from build123d import *

# Parameters (mm, degrees)
PAD_DEPTH       = 80
POCKET_DEPTH    = 78
POCKET001_DEPTH = 408.7079232475
POCKET002_DEPTH = 408.4326470939
SKETCH004_W     = 433.609177
SKETCH004_H     = 149.2376851805
SKETCH004_W_2   = 114.034424
SKETCH004_H_2   = 150.6867891805
POCKET003_DEPTH = 80.001
SKETCH005_W     = 8
SKETCH005_H     = 8
POCKET004_DEPTH = 10
SKETCH006_W     = 8
SKETCH006_H     = 8
POCKET005_DEPTH = 10
SKETCH007_R     = 1.55
POCKET006_DEPTH = 12.001
POCKET007_DEPTH = 12.001
FILLET_R        = 2
FILLET001_R     = 2


with BuildPart() as part:
    # Sketch → Pad (new body)
    with BuildSketch(Plane.XY):
        Polygon((450, 0), (450, 90), (356, 87.18), (355.64, 99.18), (343.64, 98.82), (344, 86.82), (6, 76.68), (5.64, 88.6800000001), (-6.36, 88.3200000001), (-6, 76.32), (-50, 75), (-50, 0), align=None)
    extrude(amount=PAD_DEPTH)

    # Sketch001 (on Face14 of Pad) → Pocket (cut)
    with BuildSketch(Plane.XY.offset(80)):
        Polygon((-50, 15), (-50, 74), (450, 74), (450, 0), (356, 2.82), (356.3, 12.82), (344.3, 13.18), (344, 3.18), (6, 13.32), (6.3, 23.32), (-5.7, 23.68), (-6, 13.68), align=None)
    extrude(amount=-POCKET_DEPTH, mode=Mode.SUBTRACT)

    # Sketch002 (on Face26 of Pocket) → Pocket001 (cut, through all)
    with BuildSketch(Plane(origin=(355.5953641722, -10.6678609252, 0), x_dir=(0.0299865091, 0.9995503035, 0), z_dir=(0.9995503035, -0.0299865091, 0))):
        with BuildLine():
            ThreePointArc((23.4984280855, 56), (19.9988591841, 57.4495689014), (21.4484280855, 53.95))
            ThreePointArc((21.4484280855, 53.95), (17.8329435114, 41), (21.4484280855, 28.05))
            ThreePointArc((21.4484280855, 28.05), (19.9988591841, 24.5504310986), (23.4984280855, 26))
            Line((23.4984280855, 26), (23.4984280855, 56))
        make_face()
    extrude(amount=-POCKET001_DEPTH, mode=Mode.SUBTRACT)

    # Sketch003 (on Face14 of Pocket001) → Pocket002 (cut, through all)
    with BuildSketch(Plane(origin=(358.2929363573, 10.7487880907, 0), x_dir=(-0.0299865091, 0.9995503035, 0), z_dir=(0.9995503035, 0.0299865091, 0))):
        with BuildLine():
            ThreePointArc((88.470997005, 56), (84.9714281036, 57.4495689014), (86.420997005, 53.95))
            ThreePointArc((86.420997005, 53.95), (82.8055124309, 41), (86.420997005, 28.05))
            ThreePointArc((86.420997005, 28.05), (84.9714281036, 24.5504310986), (88.470997005, 26))
            Line((88.470997005, 26), (88.470997005, 56))
        make_face()
    extrude(amount=-POCKET002_DEPTH, mode=Mode.SUBTRACT)

    # Sketch004 (on Face7 of Pocket002) → Pocket003 (cut, through all)
    with BuildSketch(Plane.XY.offset(80)):
        with Locations((127.1954115, 57.2464115903)):
            Rectangle(SKETCH004_W, SKETCH004_H)
        with Locations((413.017212, 56.5218595903)):
            Rectangle(SKETCH004_W_2, SKETCH004_H_2)
    extrude(amount=-POCKET003_DEPTH, mode=Mode.SUBTRACT)

    # Sketch005 (on Face8 of Pocket003) → Pocket004 (cut)
    with BuildSketch(Plane.XY.offset(80)):
        with Locations((350, 88)):
            Rectangle(SKETCH005_W, SKETCH005_H)
        with Locations((350, 6)):
            Rectangle(SKETCH005_W, SKETCH005_H)
    extrude(amount=-POCKET004_DEPTH, mode=Mode.SUBTRACT)

    # Sketch006 (on Face1 of Pocket004) → Pocket005 (cut)
    with BuildSketch(Plane(origin=(0, 0, 0), x_dir=(1, 0, 0), z_dir=(0, 0, -1))):
        with Locations((350, -6)):
            Rectangle(SKETCH006_W, SKETCH006_H)
        with Locations((350, -88)):
            Rectangle(SKETCH006_W, SKETCH006_H)
    extrude(amount=-POCKET005_DEPTH, mode=Mode.SUBTRACT)

    # Sketch007 (on Face6 of Pocket005) → Pocket006 (cut, through all)
    with BuildSketch(Plane.YZ.offset(356)):
        with Locations((6, 74)):
            Circle(SKETCH007_R)
        with Locations((88, 74)):
            Circle(SKETCH007_R)
        with Locations((88, 8)):
            Circle(SKETCH007_R)
        with Locations((6, 8)):
            Circle(SKETCH007_R)
    extrude(amount=-POCKET006_DEPTH, mode=Mode.SUBTRACT)

    # Sketch008 (on Face6 of Pocket006) → Pocket007 (cut, through all)
    with BuildSketch(Plane.YZ.offset(356)):
        Polygon((80, 2), (119.955566, 2), (119.955566, -12.384934), (-14.175961, -12.384934), (-14.175961, 94.92028), (80, 94.92028), (80, 65), (85, 59), (85, 23), (80, 17), align=None)
    extrude(amount=-POCKET007_DEPTH, mode=Mode.SUBTRACT)

    # Fillet
    fillet_edges = [part.edges().sort_by_distance(p)[0] for p in [
        (356, 85, 41),
    ]]
    fillet(fillet_edges, radius=FILLET_R)

    # Fillet001
    fillet001_edges = [part.edges().sort_by_distance(p)[0] for p in [
        (356, 82.5, 20),
        (356, 82.5, 62),
    ]]
    fillet(fillet001_edges, radius=FILLET001_R)


solid = part.part
The listing builds one solid part. Answer for the finished solid, in the listing's coordinates (mm). A direction names the side the tool comes from. Round coordinates to 2 decimals unless told otherwise and drop trailing zeros. Order: outer loops, then holes, each group sorted by start corner. A loop starts at its lowest first (then second) coordinate and runs counter-clockwise, first axis right, second up. Notation, with made-up numbers: (-23, 6.25) -> (24, 6.25) arc R15 ccw to (24, 25.25) -> close; hole circle Ø6 at (74, -4). An arc over 180 degrees is marked (long way). One line per item, written item: value.
Item 1: Straight lines are drawn through the part: L1, parallel to Z at x = 344.65, y = 88; L2, parallel to Z at x = 352, y = 87.75; L3, parallel to Y at x = 345.1, z = 74. For each, find the intervals that lie inside material, in ascending order.
Taken from the geometry:
L1: z = 2 to 6.45, 9.55 to 72.45, 75.55 to 80
L2: z = 10 to 70
L3: y = 80 to 86.45, 89.55 to 98.86
Item 2: Find section A-A, the plane z = 8. Give the vertices of the cut face in (x, y), then the cut area to 3 significant figures.
Taken from the geometry:
outline: (344, 80) -> (356, 80) -> (356, 86.45) -> (354, 86.45) -> (354, 84) -> (346, 84) -> (346, 86.45) -> (344, 86.45) -> close; (344, 89.55) -> (346, 89.55) -> (346, 92) -> (354, 92) -> (354, 89.55) -> (355.93, 89.55) -> (355.64, 99.18) -> (344, 98.83) -> close
area: 150 mm2
Item 3: Find section C-C, the plane z = 45. Give the vertices of the cut face in (x, y).
Taken from the geometry:
outline: (344, 85) -> (354, 85) arc R2 ccw to (356, 87) -> (356, 87.18) -> (355.8, 93.84) -> (344, 93.48) -> close
Item 4: Given P1, Ø3, axis at x = 355, z = 20.5, coming from the -Y side; P2, Ø4, axis at x = 352, z = 6.5, coming from the +Y side; P3, Ø10, axis at y = 82.5, z = 38, coming from the -X side; P4, Ø2, axis at x = 350.5, z = 34, coming from the -Y side, each flat-ended and moving along its own axis, determine where each tip first touches the part or whether it passes through.
Taken from the geometry:
P1: stops at y = 81.82
P2: stops at y = 99.13
P3: stops at x = 344
P4: stops at y = 85
Item 5: Find section B-B, the plane y = 88.25. Give the vertices of the cut face in (x, z).
Taken from the geometry:
outline: (344, 2) -> (346, 2) -> (346, 6.47) -> (344, 6.47) -> close; (344, 9.53) -> (346, 9.53) -> (346, 10) -> (354, 10) -> (354, 9.53) -> (355.97, 9.53) -> (355.97, 72.47) -> (354, 72.47) -> (354, 70) -> (346, 70) -> (346, 72.47) -> (344, 72.47) -> close; (344, 75.53) -> (346, 75.53) -> (346, 80) -> (344, 80) -> close; (354, 2) -> (355.97, 2) -> (355.97, 6.47) -> (354, 6.47) -> close; (354, 75.53) -> (355.97, 75.53) -> (355.97, 80) -> (354, 80) -> close
Item 6: For faces 5 (the cylindrical face through (349.94, 95.46, 24.6)), 6 (the flat face through (349.1, 82.5, 62)), 7 (the flat face through (350, 84, 6)), 8 (the flat face through (350, 84, 75)), 9 (the cylindrical face through (355.4, 82.45, 62.95)), determine the directions among +Z, -Z, +X, -X, +Y, -Y from which every point of the face is accessible in a straight line to the end or side of a thin tool.
Taken from the geometry:
face 5: none
face 6: +X, -X, -Y
face 7: -Z
face 8: +Z
face 9: +X, -Y
Item 7: For a pull along X with two mould halves and no side action, classify faces 1 (the cylindrical face through (355.4, 82.45, 19.05)), 2 (the cylindrical face through (345.014, 89.478, 8.466)), 3 (the flat face through (350, 92, 75)), 4 (the flat face through (346, 88, 6)) as released by +X, released by -X, zero draft, split by the parting line, or undercut.
Taken from the geometry:
face 1: released by +X
face 2: zero draft
face 3: undercut
face 4: undercut
